Design review of the part built by this model. Coordinates are the model's own, in mm. Face numbers are marked on the shaded views. A direction names the side the tool comes from. Coordinates: 2 decimals unless noted, no trailing zeros. Order: outer loops, then holes, each group sorted by start corner. A loop starts at its lowest first (then second) coordinate and runs counter-clockwise, first axis right, second up. Notation, with made-up numbers: (-35, -10.5) -> (-10, -10.5) arc R18 ccw to (-10, 6.5) -> close; hole circle Ø4 at (58, 5). An arc over 180 degrees is marked (long way). Use a Markdown table: item, result. Add a question column.
Q1. Add section C-C (y = -4.5). State the section outline as (x, z) points, then the cut area to 3 significant figures.
Q2. Add section A-A (z = 0). State the section outline as (x, y) points.
Q3. The part is to be moulded in two halves that separate along Y. For the marked faces 3, 4 and 5, say which applies: pulls with the +Y half, pulls with the -Y half, needs draft (parallel to the pull), parting line crosses it, or undercut.
Q4. Wall thickness on probe 1 along Z at (x, y) = (0, -4.25); probe 2 along Z at (x, y) = (0, -0.25); probe 3 along Y at (x, z) = (0, -6.95): over which ranges is each line inside the solid? List them lowest first.
Q5. Insertion check: pin 1 (6 mm diameter, centred on y = 1.5, z = -5, fed in from +X); pin 2 (1 mm diameter, centred on x = 3, y = -7, fed in from +Z); pin 3 (4 mm diameter, centred on y = -6, z = 7, fed in from -X). Each pin has a flat end and moves straight along its axis. Give the tip position at first contact, or say it passes through.
Q6. Add section B-B (x = 0). State the section outline as (y, z) points, then the cut area to 3 significant figures.
Q7. Machinability: for the marked faces 1 and 2, which of the approach directions +Z, -Z, +X, -X, +Y, -Y give a long, thin tool a straight path to every point of the face, cutting with its end or side? Answer none if there is none.
Q8. Add section D-D (z = 3.5). State the section outline as (x, y) points.
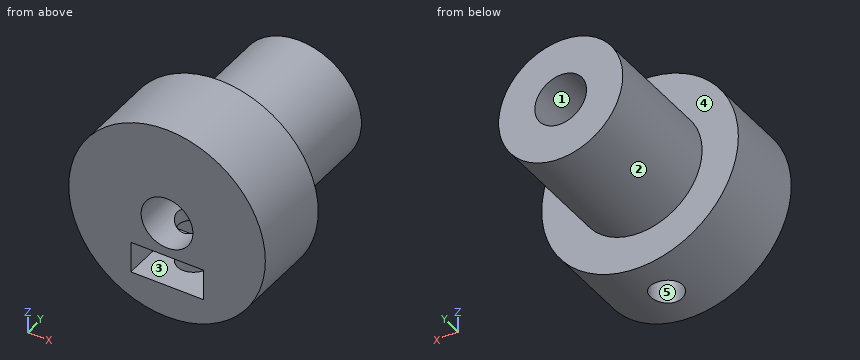
Autodesk Inventor part; units mm, degrees
ref_plane "YZ Plane" through (0, 0, 0) normal (1, 0, 0) x (0, 1, 0)
ref_plane "XZ Plane" through (0, 0, 0) normal (0, 1, 0) x (-1, 0, 0)
ref_plane "XY Plane" through (0, 0, 0) normal (0, 0, 1) x (1, 0, 0)
sketch "Sketch1" plane through (0, 0, 0) normal (0, 1, 0) x (-1, 0, 0)
  circle A0 centre (0, 0) radius 6
  dimension "d0" = 12
extrude "Extrusion1" add sketch "Sketch1" along normal blind 9 and the other way blind 3
sketch "Sketch2" plane through (0, -3, 0) normal (0, -1, 0) x (1, 0, 0)
  circle A0 centre (0, 0) radius 9.5
  dimension "d3" = 19
extrude "Extrusion2" add sketch "Sketch2" along normal blind 8
sketch "Sketch7" plane through (0, 0, 0) normal (0, 0, 1) x (1, 0, 0)
  point P0 (0, 0)
sketch "Sketch9" plane through (0, 0, 0) normal (0, 0, 1) x (1, 0, 0)
  circle A0 centre (0, -7) radius 1.55
  line L0 (-9.5, -11) -> (9.5, -11)
  line L1 (0, -11) -> (0, -3)
  line L2 (0, -11) -> (0, -3)
  line L3 (-6, -3) -> (6, -3)
  point P0 (0, 0)
  point P1 (0, -7)
  dimension "d22" = 3.1
extrude "Extrusion8" cut sketch "Sketch9" against normal up to next
sketch "Sketch10" plane through (0, 9, 0) normal (0, 1, 0) x (1, 0, 0)
  circle A0 centre (0, 0) radius 2.5
  dimension "d26" = 5
extrude "Extrusion9" cut sketch "Sketch10" against normal through all
sketch "Sketch11" plane through (0, -11, 0) normal (0, -1, 0) x (1, 0, 0)
  line L0 (3.5, -6.3359) -> (-3.5, -6.3359)
  line L1 (-3.5, -6.3359) -> (-3.5, -3.3359)
  line L2 (-3.5, -3.3359) -> (3.5, -3.3359)
  line L3 (3.5, -3.3359) -> (3.5, -6.3359)
  circle A0 centre (0, 0) radius 9.5
  circle A1 centre (0, 0) radius 2.5
  point P0 (0, -3.3359)
  dimension "d29" = 7
  dimension "d30" = 3
extrude "Extrusion10" cut sketch "Sketch11" against normal blind 7 contours L0 L1 L2 L3
properties part number "штука от моторчика2015" material "Bronze, Cast"
Established:
| question | item | result |
|---|---|---|
| 1 | outline | circle Ø19 at (0, 0); hole (-3.5, -6.34) -> (3.5, -6.34) -> (3.5, -3.34) -> (-3.5, -3.34) -> close; hole circle Ø5 at (0, 0) |
| 1 | area | 243 mm^2 |
| 2 | outline | (-9.5, -11) -> (-2.5, -11) -> (-2.5, 9) -> (-6, 9) -> (-6, -3) -> (-9.5, -3) -> close; (2.5, -11) -> (9.5, -11) -> (9.5, -3) -> (6, -3) -> (6, 9) -> (2.5, 9) -> close |
| 3 | face 3 | needs draft |
| 3 | face 4 | pulls with the +Y half |
| 3 | face 5 | undercut |
| 4 | probe 1 | -9.5 to -6.34, -3.34 to -2.5, 2.5 to 9.5 |
| 4 | probe 2 | -6 to -2.5, 2.5 to 6 |
| 4 | probe 3 | -11 to -8.55, -5.45 to -3 |
| 5 | pin 1 | x = 5.66 |
| 5 | pin 2 | z = 9.17 |
| 5 | pin 3 | x = -8.08 |
| 6 | outline | (-11, -9.5) -> (-8.55, -9.5) -> (-8.55, -6.34) -> (-11, -6.34) -> close; (-11, -3.34) -> (-8.55, -3.34) -> (-8.55, -2.5) -> (-11, -2.5) -> close; (-11, 2.5) -> (9, 2.5) -> (9, 6) -> (-3, 6) -> (-3, 9.5) -> (-11, 9.5) -> close; (-5.45, -9.5) -> (-3, -9.5) -> (-3, -6) -> (9, -6) -> (9, -2.5) -> (-5.45, -2.5) -> (-5.45, -3.34) -> (-4, -3.34) -> (-4, -6.34) -> (-5.45, -6.34) -> close |
| 6 | area | 163 mm^2 |
| 7 | face 1 | +Y, -Y |
| 7 | face 2 | +Y |
| 8 | outline | (-8.83, -11) -> (8.83, -11) -> (8.83, -3) -> (4.87, -3) -> (4.87, 9) -> (-4.87, 9) -> (-4.87, -3) -> (-8.83, -3) -> close |
